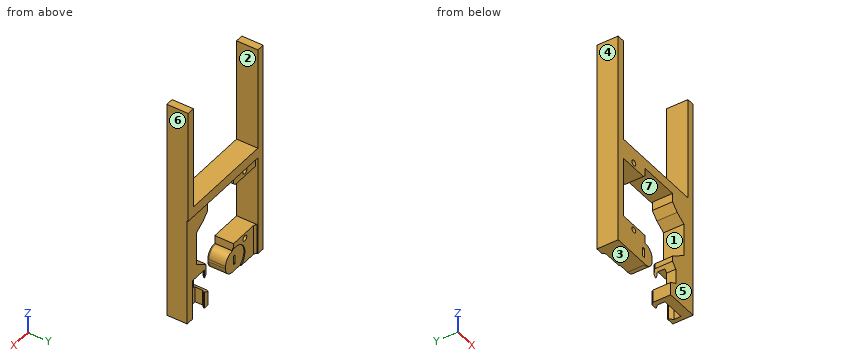
from build123d import *
from OCP.BRepFilletAPI import BRepFilletAPI_MakeChamfer

# Parameters (mm, degrees)
SKETCH1_W                       = 3
SKETCH1_H                       = 37
SKETCH1_H_2                     = 48
BOSS_EXTRUDE1_DEPTH             = 8
SKETCH4_W                       = 19.5
SKETCH4_H                       = 8.8
BOSS_EXTRUDE3_DEPTH             = 6.6
SERVO_HOLDER_DEPTH              = 0.4
SERVO_HOLDER_DEPTH_BACK         = 7
SKETCH3_W                       = 15.5
SKETCH3_H                       = 4
SKETCH3_R                       = 1.04
SKETCH5_W                       = 1
SKETCH5_H                       = 3.6
CUT_EXTRUDE2_DEPTH              = 70.647801738
SKETCH11_W                      = 43
SKETCH11_H                      = 4
BOSS_EXTRUDE9_DEPTH             = 8
BOSS_EXTRUDE9_DIRECTION_2_REACH = 71.601
SKETCH14_W                      = 12.223643904
SKETCH14_H                      = 44.979564252
CUT_EXTRUDE5_DEPTH              = 10
FILLET2_R                       = 3.9
CUT_EXTRUDE4_DEPTH              = 70.647801738
CUT_EXTRUDE4_DEPTH_BACK         = 70.647801738
SKETCH13_R                      = 1.1
SKETCH17_W                      = 12.9
SKETCH17_H                      = 8
BOSS_EXTRUDE11_DEPTH            = 27
BOSS_EXTRUDE12_DEPTH            = 16
SKETCH18_W                      = 1
SKETCH18_H                      = 3.6
SKETCH18_W_2                    = 3
SKETCH18_H_2                    = 24
SKETCH18_H_3                    = 41
BOSS_EXTRUDE13_DEPTH            = 0.4
CHAMFER14_SIZE                  = 1.2
CUT_EXTRUDE6_DEPTH              = 73.439806169
CUT_EXTRUDE6_DEPTH_BACK         = 73.439806169
SKETCH29_W                      = 8.885937164
SKETCH29_H                      = 8
BOSS_EXTRUDE20_DEPTH            = 0.4
CHAMFER23_SIZE                  = 1
CHAMFER24_SIZE                  = 1
CHAMFER24_SIZE2                 = 3.099667104
SKETCH26_R                      = 5.5
CUT_EXTRUDE8_DEPTH              = 10
CHAMFER25_SIZE                  = 0.6
CHAMFER25_SIZE2                 = 1.039230485


with BuildPart() as part:
    # Sketch1 → Boss-Extrude1 (new body)
    with BuildSketch(Plane(origin=(0, 0, 0), x_dir=(1, 0, 0), z_dir=(0, 1, 0))):
        with Locations((-20, -0.788461538)):
            Rectangle(SKETCH1_W, SKETCH1_H)
        with Locations((-20, 41.711538462)):
            Rectangle(SKETCH1_W, SKETCH1_H_2)
        with Locations((20, -0.788461538)):
            Rectangle(SKETCH1_W, SKETCH1_H)
        with Locations((20, 41.711538462)):
            Rectangle(SKETCH1_W, SKETCH1_H_2)
    extrude(amount=-BOSS_EXTRUDE1_DEPTH)

    # Sketch4 → Boss-Extrude3 (add)
    with BuildSketch(Plane.XZ.offset(8)):
        with Locations((-11.75, -61.311538462)):
            Rectangle(SKETCH4_W, SKETCH4_H)
    extrude(amount=-BOSS_EXTRUDE3_DEPTH)

    # Sketch3 → Servo Holder (add, two sides: drawn at the far end of the back side and taken through both)
    # profile 1 of 2: a face of its own
    with BuildSketch(Plane.XZ.offset(8).offset(-SERVO_HOLDER_DEPTH_BACK)):
        with Locations((-13.75, -55.711538462)):
            Rectangle(SKETCH3_W, SKETCH3_H)
        with Locations(Location((-12.5, -55.711538462, 0), (0, 0, 270))):
            Circle(SKETCH3_R, mode=Mode.SUBTRACT)
    # profile 2 of 2: a face of its own
    with BuildSketch(Plane.XZ.offset(8).offset(-SERVO_HOLDER_DEPTH_BACK)):
        with Locations((-13.75, -27.711538462)):
            Rectangle(SKETCH3_W, SKETCH3_H)
        with Locations(Location((-12.5, -27.711538462, 0), (0, 0, 90))):
            Circle(SKETCH3_R, mode=Mode.SUBTRACT)
    extrude(amount=SERVO_HOLDER_DEPTH + SERVO_HOLDER_DEPTH_BACK)

    # Sketch5 → Cut-Extrude2 (cut, through all)
    with BuildSketch(Plane(origin=(0, 0, 0), x_dir=(1, 0, 0), z_dir=(0, 1, 0))):
        with Locations((-7, 61.311538462)):
            Rectangle(SKETCH5_W, SKETCH5_H)
    extrude(amount=-CUT_EXTRUDE2_DEPTH, mode=Mode.SUBTRACT)

    # Sketch11 → Boss-Extrude9 (add)
    with BuildSketch(Plane.XZ.offset(8)):
        with Locations((0, -23.711538462)):
            Rectangle(SKETCH11_W, SKETCH11_H)
    extrude(amount=-BOSS_EXTRUDE9_DEPTH)

    # Boss-Extrude9 direction 2: up to this face of the body (flat: up to its plane)
    boss_extrude9_direction_2_end = Plane(part.part.faces().sort_by_distance((-13.822479257, -8.4, -55.711538462))[0])
    # Sketch11 → Boss-Extrude9 direction 2 (add, up to the picked face)
    with BuildSketch(Plane.XZ.offset(8), mode=Mode.PRIVATE) as boss_extrude9_direction_2_sk1:
        with Locations((0, -23.711538462)):
            Rectangle(SKETCH11_W, SKETCH11_H)
    boss_extrude9_direction_2_tool1 = split(extrude(boss_extrude9_direction_2_sk1.sketch, amount=BOSS_EXTRUDE9_DIRECTION_2_REACH, mode=Mode.PRIVATE), bisect_by=boss_extrude9_direction_2_end, keep=Keep.BOTH, mode=Mode.PRIVATE)
    add(boss_extrude9_direction_2_tool1.solids().sort_by(Axis((0, -8, -23.711538), (0, -1, 0)))[0])

    # Sketch14 → Cut-Extrude5 (cut)
    with BuildSketch(Plane.XZ.offset(8)):
        with Locations((24.611821952, -48.201320588)):
            Rectangle(SKETCH14_W, SKETCH14_H)
    extrude(amount=-CUT_EXTRUDE5_DEPTH, mode=Mode.SUBTRACT)

    # Fillet2
    fillet2_edges = [part.edges().sort_by_distance(p)[0] for p in [
        (-2, -4.7, -65.711538462),
        (-2, -4.7, -56.911538462),
    ]]
    fillet(fillet2_edges, radius=FILLET2_R)

    # Sketch13 → Cut-Extrude4 (cut, two sides: drawn at the far end of the back side and taken through both)
    with BuildSketch(Plane(origin=(0, -8.4, 0), x_dir=(-1, 0, 0), z_dir=(0, -1, 0)).offset(-CUT_EXTRUDE4_DEPTH_BACK)):
        with Locations(Location((12.5, 55.711538462, 0), (0, 0, 270))):
            Circle(SKETCH13_R)
        with Locations(Location((12.5, 27.711538462, 0), (0, 0, 270))):
            Circle(SKETCH13_R)
    extrude(amount=CUT_EXTRUDE4_DEPTH + CUT_EXTRUDE4_DEPTH_BACK, mode=Mode.SUBTRACT)

    # Sketch17 → Boss-Extrude11 (add)
    with BuildSketch(Plane(origin=(0, 0, -25.711538462), x_dir=(-1, 0, 0), z_dir=(0, 0, -1))):
        with Locations((-15.05, -4.4)):
            Rectangle(SKETCH17_W, SKETCH17_H)
    extrude(amount=BOSS_EXTRUDE11_DEPTH)

    # Sketch16 → Boss-Extrude12 (add)
    with BuildSketch(Plane(origin=(0, 0, -52.711538462), x_dir=(-1, 0, 0), z_dir=(0, 0, -1))):
        Polygon((-19.75, -2), (-18.55, -2), (-18.55, -0.4), (-21.5, -0.4), (-21.5, -8.4), (-8.6, -8.4), (-8.6, -0.4), (-11.55, -0.4), (-11.55, -2), (-10.55, -2), (-10.55, -4.8), (-19.75, -4.8), align=None)
    extrude(amount=BOSS_EXTRUDE12_DEPTH)

    # Sketch18 → Boss-Extrude13 (add)
    # profile 1 of 4: a face of its own
    with BuildSketch(Plane.XZ.offset(8)):
        with BuildLine():
            Line((-21.5, -57.711538462), (-21.5, -65.711538462))
            Line((-21.5, -65.711538462), (-5.9, -65.711538462))
            ThreePointArc((-5.9, -65.711538462), (-3.142283553, -64.569254908), (-2, -61.811538462))
            Line((-2, -61.811538462), (-2, -60.811538462))
            ThreePointArc((-2, -60.811538462), (-3.142283553, -58.053822015), (-5.9, -56.911538462))
            Line((-5.9, -56.911538462), (-6, -56.911538462))
            Line((-6, -56.911538462), (-6, -57.711538462))
            Line((-6, -57.711538462), (-21.5, -57.711538462))
        make_face()
        with Locations((-7, -61.311538462)):
            Rectangle(SKETCH18_W, SKETCH18_H, mode=Mode.SUBTRACT)
    # profile 2 of 4: a face of its own
    with BuildSketch(Plane.XZ.offset(8)):
        with Locations((-20, -41.711538462)):
            Rectangle(SKETCH18_W_2, SKETCH18_H_2)
    # profile 3 of 4: a face of its own
    with BuildSketch(Plane.XZ.offset(8)):
        with Locations((-20, -1.211538462)):
            Rectangle(SKETCH18_W_2, SKETCH18_H_3)
    # profile 4 of 4: a face of its own
    with BuildSketch(Plane.XZ.offset(8)):
        with Locations((20, -1.211538462)):
            Rectangle(SKETCH18_W_2, SKETCH18_H_3)
    extrude(amount=BOSS_EXTRUDE13_DEPTH)

    # Chamfer14
    # the kernel refuses this chamfer: 1.2 mm, written as the material it takes off along each edge
    with BuildSketch(Plane(origin=(18.55, -2, -52.711538462), x_dir=(0.9996219169112968, -0.027495876610586622, 0), z_dir=(0, 0, -1))) as chamfer14_piece_1_section:
        Polygon((CHAMFER14_SIZE * 0.999621916911, -CHAMFER14_SIZE * 0.0274958766106), (-CHAMFER14_SIZE * 0.0274958766106, -CHAMFER14_SIZE * 0.999621916911), (0, 0), align=None)
    chamfer14_piece_1 = extrude(amount=19.086019586, mode=Mode.PRIVATE)
    chamfer14_piece_1 = split(chamfer14_piece_1, bisect_by=Plane(origin=(19.75, -1.603515015, -62.254548254), z_dir=(-1, 0, 0)), keep=Keep.TOP, mode=Mode.PRIVATE)
    add(chamfer14_piece_1, mode=Mode.SUBTRACT)
    with BuildSketch(Plane(origin=(11.55, -2, -52.711538462), x_dir=(0.027495876610585914, 0.9996219169112968, 0), z_dir=(0, 0, -1))) as chamfer14_piece_2_section:
        Polygon((CHAMFER14_SIZE * 0.999621916911, -CHAMFER14_SIZE * 0.0274958766106), (-CHAMFER14_SIZE * 0.0274958766106, -CHAMFER14_SIZE * 0.999621916911), (0, 0), align=None)
    chamfer14_piece_2 = extrude(amount=19.086019586, mode=Mode.PRIVATE)
    chamfer14_piece_2 = split(chamfer14_piece_2, bisect_by=Plane(origin=(10.55, -1.589568171, -62.254548254), z_dir=(1, 0, 0)), keep=Keep.TOP, mode=Mode.PRIVATE)
    add(chamfer14_piece_2, mode=Mode.SUBTRACT)

    # Sketch20 → Cut-Extrude6 (cut, two sides: drawn at the far end of the back side and taken through both)
    with BuildSketch(Plane(origin=(0, -0.4, 0), x_dir=(1, 0, 0), z_dir=(0, 1, 0)).offset(-CUT_EXTRUDE6_DEPTH_BACK)):
        Polygon((8.6, 53.963605621), (8.6, 63.570761525), (2.515498959, 66.765310983), (1.997773223, 58.659131413), (1.997773223, 53.963605621), (4.974693998, 53.963605621), (4.974693998, 55.162371456), (6.687222193, 53.963605621), align=None)
        Polygon((8.6, 52.700948092), (8.6, 53.963605621), (6.687222193, 53.963605621), (8.558718605, 52.653562397), align=None)
        Polygon((16.174786864, 47.322331969), (9.7, 51.854668021), (9.7, 30.195176122), (16.174786864, 34.211808124), align=None)
        Polygon((4.974693998, 53.963605621), (6.687222193, 53.963605621), (4.974693998, 55.162371456), align=None)
        Polygon((11.55, 56.087166011), (11.55, 62.021921145), (8.6, 63.570761525), (8.6, 53.963605621), (9.7, 53.963605621), align=None)
        Polygon((8.6, 52.624665515), (8.6, 52.700948092), (8.558718605, 52.653562397), align=None)
        Polygon((9.7, 25.711538462), (9.7, 30.195176122), (8.6, 29.512791467), (8.6, 25.711538462), align=None)
        Polygon((9.7, 53.963605621), (8.6, 53.963605621), (8.6, 52.700948092), align=None)
        Polygon((9.7, 51.854668021), (9.7, 53.963605621), (8.6, 52.700948092), (8.6, 52.624665515), align=None)
        Polygon((8.558718605, 52.653562397), (6.687222193, 53.963605621), (4.974693998, 53.963605621), (4.974693998, 48.539566347), align=None)
        Polygon((9.7, 30.195176122), (9.7, 51.854668021), (8.6, 52.624665515), (8.6, 29.512791467), align=None)
        Polygon((8.6, 52.624665515), (8.558718605, 52.653562397), (4.974693998, 48.539566347), (4.974693998, 27.263834025), (8.6, 29.512791467), align=None)
    extrude(amount=CUT_EXTRUDE6_DEPTH + CUT_EXTRUDE6_DEPTH_BACK, mode=Mode.SUBTRACT)

    # Sketch29 → Boss-Extrude20 (add)
    with BuildSketch(Plane(origin=(0, -1.4, 0), x_dir=(1, 0, 0), z_dir=(0, 1, 0))):
        with Locations((-14.057031418, 61.711538462)):
            Rectangle(SKETCH29_W, SKETCH29_H)
    extrude(amount=BOSS_EXTRUDE20_DEPTH)

    # Chamfer23
    chamfer23_edges = [part.edges().sort_by_distance(p)[0] for p in [
        (9.7, -0.4, -52.909136821),
    ]]
    chamfer(chamfer23_edges, length=CHAMFER23_SIZE)

    # Chamfer24: one chamfer whose edges measure the first distance from different faces: ONE call of the kernel's chamfer builder (chamfer() names one face for all edges)
    chamfer24_edges_1 = [part.edges().sort_by_distance(p)[0] for p in [
        (8.6, -0.4, -66.141149993),
        (-6, -4.7, -29.711538462),
    ]]
    chamfer24_edges_2 = [part.edges().sort_by_distance(p)[0] for p in [
        (9.7, -4.4, -30.195176122),
    ]]
    chamfer24_side_2 = [part.faces().sort_by_distance(p)[0] for p in [
        (9.7, -4.4, -27.953357292),
    ]]
    chamfer24 = BRepFilletAPI_MakeChamfer(part.part.solid().wrapped)
    for e in chamfer24_edges_1:
        chamfer24.Add(CHAMFER24_SIZE, e.wrapped)
    for e in chamfer24_edges_2:
        chamfer24.Add(CHAMFER24_SIZE, CHAMFER24_SIZE2, e.wrapped, chamfer24_side_2[0].wrapped)  # the first distance lies on this face
    add(Compound.cast(chamfer24.Shape()), mode=Mode.REPLACE)

    # Sketch26 → Cut-Extrude8 (cut)
    with BuildSketch(Plane(origin=(0, -1.4, 0), x_dir=(1, 0, 0), z_dir=(0, 1, 0))):
        with Locations((-7, 61.311538462)):
            Circle(SKETCH26_R)
    extrude(amount=CUT_EXTRUDE8_DEPTH, mode=Mode.SUBTRACT)

    # Chamfer25
    chamfer25_edges = [part.edges().sort_by_distance(p)[0] for p in [
        (-18.5, -1, -59.711538462),
    ]]
    chamfer25_side = [part.faces().sort_by_distance(p)[0] for p in [
        (-18.5, -3.927941176, -42.446832579),
    ]]
    chamfer(chamfer25_edges, length=CHAMFER25_SIZE, length2=CHAMFER25_SIZE2, reference=chamfer25_side[0])


solid = part.part
Read the model definition and answer for the solid it produces. Units are mm, in the model's axes. Face numbers are marked on the shaded views. A direction names the side the tool comes from. Round coordinates to 2 decimals unless told otherwise and drop trailing zeros. Loops run counter-clockwise (first coordinate to the right, second up) from the corner with the lowest first, then second, coordinate; pieces in that order, holes last.
Q1. Determine the mould class of the marked faces 5, 6 and 7 for opening direction X: released by +X, released by -X, zero draft, split by the parting line, or undercut.
Q2. Section A-A on x = 17 is taken. Write down the section's boundary in (y, z).
Q3. Each of these flat-tipped pins is pushed along its axis until it touches: pin 1 (6 mm diameter, centred on x = 15, z = -39, fed in from +Y); pin 2 (1.1 mm diameter, centred on x = -7, y = -6, fed in from -Z); pin 3 (9 mm diameter, centred on x = -10, z = -59, fed in from +Y). Where does it stop, or does it pass through?
Q4. Section D-D on x = 7 is taken. Write down the section's boundary in (y, z).
Q5. Section C-C on y = -6.75 is taken. Give the number of separate pieces and of enclosed holes in the cut face, and give its area (3 significant figures).
Q6. Consider probe 1 along X at (y, z) = (-6, -27.5); probe 2 along X at (y, z) = (-7.5, -42); probe 3 along X at (y, z) = (-7, -28.5). Determine where each line is inside the solid, lowest interval first.
Q7. Section B-B on z = -10.5 is taken. Write down the section's boundary in (x, y).
Q8. Which of the six approach directions +Z, -Z, +X, -X, +Y, -Y give full straight-line access (tool end or side, diameter ignored) to the marked faces 1, 2, 3 and 4?
Output:
1. face 5: zero draft
1. face 6: released by +X
1. face 7: undercut
2. outline: (-8.4, -68.71) - (-4.8, -68.71) - (-4.8, -52.71) - (-0.4, -52.71) - (-0.4, -25.71) - (0, -25.71) - (0, -21.71) - (-8.4, -21.71) - close
3. pin 1: stops at y = -0.4
3. pin 2: stops at z = -65.71
3. pin 3: stops at y = -1
4. outline: (-8.4, -25.71) - (0, -25.71) - (0, -21.71) - (-8.4, -21.71) - close
5. separate pieces: 1
5. enclosed holes: 3
5. area: 1,140 mm2
6. probe 1: x = -21.5 to -13.58, -11.42 to -6, 9.7 to 21.5
6. probe 2: x = -21.5 to -18.5, 16.17 to 21.5
6. probe 3: x = -21.5 to -13.27, -11.73 to -6, 9.7 to 21.5
7. outline: (-21.5, -8.4) - (-18.5, -8.4) - (-18.5, 0) - (-21.5, 0) - close; (18.5, -8.4) - (21.5, -8.4) - (21.5, 0) - (18.5, 0) - close
8. face 1: +Y, -Y
8. face 2: +Z, +Y, -Y
8. face 3: -Z, -X, +Y, -Y
8. face 4: +Z, -Z, -X, +Y, -Y
